```python
from build123d import *

# Parameters (mm, degrees)
SKETCH_1_R      = 8
SKETCH_1_R_2    = 5
EXTRUDE_1_DEPTH = 6
CHAMFER_1_SIZE  = 1


with BuildPart() as part:
    # Эскиз1 → Вытянуть1 (new body)
    with BuildSketch(Plane.XY):
        Circle(SKETCH_1_R)
        Circle(SKETCH_1_R_2, mode=Mode.SUBTRACT)
    extrude(amount=EXTRUDE_1_DEPTH)

    # Фаска1
    chamfer_1_edges = [part.edges().sort_by_distance(p)[0] for p in [
        (-8, 0, 6),
    ]]
    chamfer(chamfer_1_edges, length=CHAMFER_1_SIZE)

    # Эскиз4 → Вырез-Повернуть1 (revolve, cut)
    with BuildSketch(Plane(origin=(0, 0, 0), x_dir=(0, 0, -1), z_dir=(1, 0, 0)), mode=Mode.PRIVATE) as cut_revolve_1_sk:
        Polygon((0, 8), (-6, 7.76), (-6, 8), align=None)
    revolve(cut_revolve_1_sk.sketch.rotate(Axis((0, 0, 6), (0, 0, -1)), 90), axis=Axis((0, 0, 6), (0, 0, -1)), mode=Mode.SUBTRACT)


solid = part.part
```
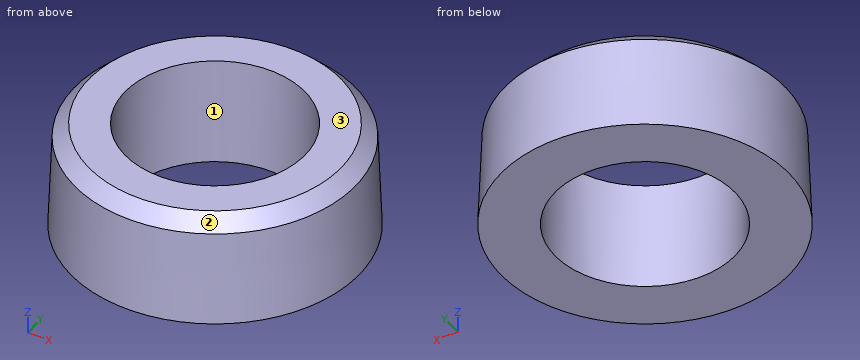
Verification items for the finished model (mm, model axes). Face numbers are marked on the shaded views. Coordinates: 2 decimals unless noted, no trailing zeros. Write each loop counter-clockwise with the first axis right and the second up, starting at its lowest first coordinate (ties: lowest second). Pieces come first, ordered by that corner, then holes. Notation, with made-up numbers: M -20.75,-8 L 33.25,-8 A32 ccw 33.25,22 Z; hole C 87,-19 d3. An arc over 180 degrees is marked long. One line per item, written item: value.
Item 1: Mould release check, pull along X, two halves, no side actions. Record for the marked faces 1, 2 and 3: pulls with the +X half, pulls with the -X half, needs draft (parallel to the pull), parting line crosses it, or undercut.
Check sheet entries:
face 1: undercut
face 2: parting line crosses it
face 3: needs draft
Item 2: Section check C-C, the plane z = 2.25. Record the boundary of the cut face in (x, y), plus the area to 3 significant figures.
Check sheet entries:
outline: C 0,0 d15.82; hole C 0,0 d10
area: 118 mm^2
Item 3: Scan lines: line 1 along X through (y, z) = (0.5, 5.2); line 2 along Y through (x, z) = (0, 4.45); line 3 along X through (y, z) = (2.25, 5.1). Record each from-to range of solid material in increasing order.
Check sheet entries:
line 1: x = -7.78 to -4.97, 4.97 to 7.78
line 2: y = -7.82 to -5, 5 to 7.82
line 3: x = -7.46 to -4.47, 4.47 to 7.46
Item 4: Section check A-A, the plane y = 0. Record the boundary of the cut face in (x, z), plus the area to 3 significant figures.
Check sheet entries:
outline: M -8,0 L -5,0 L -5,6 L -7,6 L -7.79,5.21 Z; M 5,0 L 8,0 L 7.79,5.21 L 7,6 L 5,6 Z
area: 34.0 mm^2
Item 5: Gauge pin test, flat ends, axial feed: pin 1 Ø1 at (y, z) = (-0.5, 3.5) entering from -X; pin 2 Ø2 at (y, z) = (4.5, 3.5) entering from -X; pin 3 Ø2 at (y, z) = (-2.5, 3.5) entering from +X. Record the tip position at first contact, or that the pin passes through.
Check sheet entries:
pin 1: stops at x = -7.87
pin 2: stops at x = -7.04
pin 3: stops at x = 7.72
Item 6: Section check D-D, the plane z = 0.95. Record the boundary of the cut face in (x, y), plus the area to 3 significant figures.
Check sheet entries:
outline: C 0,0 d15.92; hole C 0,0 d10
area: 121 mm^2
